Geometry: final body of the model. Coordinates: model frame, mm. Face numbers are marked on the shaded views. A direction names the side the tool comes from. Coordinates: 2 decimals unless noted, no trailing zeros. Write each loop counter-clockwise with the first axis right and the second up, starting at its lowest first coordinate (ties: lowest second). Pieces come first, ordered by that corner, then holes. Notation, with made-up numbers: M -37,-10.5 L -1,-10.5 A32 cw -1,22.5 Z; hole C 8,11.5 d4. An arc over 180 degrees is marked long. Write item = value, one per line. Start each with the question number.
Item 1: Reachability of the marked faces 1 and 2 from +Z, -Z, +X, -X, +Y, -Y: full face, straight path, thin tool, end or side. Return the list, or none.
Item 2: First-contact query: pin 1 Ø2 at (x, z) = (-4.5, -1.5) entering from +Y; pin 2 Ø2 at (x, y) = (2.5, 20) entering from -Z; pin 3 Ø2 at (x, y) = (-4.5, 9) entering from +Z; pin 4 Ø5 at (x, z) = (-3, 2) entering from +Y. Flat tips, straight axial feed; report the tip coordinate or a pass-through.
Item 3: Ray query, L1, parallel to Y at x = -3, z = -1; L2, parallel to Y at x = 1.25, z = 4.75; L3, parallel to X at y = 30.5, z = -0.25. Return the intervals inside material, ascending. Write a range as [from, to].
Item 4: Section B-B on y = 39.5. Output: boundary loops of the cut face in (x, z), plus the area to 3 significant figures.
Item 5: Section A-A on x = 0. Output: boundary loops of the cut face in (y, z).
from build123d import *

# Parameters (mm, degrees)
SKETCH1_R           = 4
BOSS_EXTRUDE1_DEPTH = 65
BOSS_EXTRUDE2_DEPTH = 5
FILLET1_R           = 1
FILLET2_R           = 1


with BuildPart() as part:
    # Sketch1 → Boss-Extrude1 (new body)
    with BuildSketch(Plane(origin=(0, 0, 0), x_dir=(1, 0, 0), z_dir=(0, 1, 0))):
        with Locations(Location((0, 0, 0), (0, 0, 270))):
            Circle(SKETCH1_R)
    extrude(amount=BOSS_EXTRUDE1_DEPTH)

    # Sketch2 → Boss-Extrude2 (add)
    with BuildSketch(Plane.XZ):
        Polygon((-3.464101615, -6), (3.464101615, -6), (6.92820323, 0), (3.464101615, 6), (-3.464101615, 6), (-6.92820323, 0), align=None)
    extrude(amount=BOSS_EXTRUDE2_DEPTH)

    # Fillet1
    fillet1_edges = [part.edges().sort_by_distance(p)[0] for p in [
        (0, 65, -4),
    ]]
    fillet(fillet1_edges, radius=FILLET1_R)

    # Fillet2
    fillet2_edges = [part.edges().sort_by_distance(p)[0] for p in [
        (-5.196152423, 0, -3),
        (-6.92820323, -2.5, 0),
        (0, 0, -6),
        (-3.464101615, -2.5, -6),
        (5.196152423, 0, -3),
        (3.464101615, -2.5, -6),
        (5.196152423, 0, 3),
        (6.92820323, -2.5, 0),
        (0, 0, 6),
        (3.464101615, -2.5, 6),
        (-5.196152423, 0, 3),
        (-3.464101615, -2.5, 6),
        (-5.196152423, -5, -3),
        (0, -5, -6),
        (5.196152423, -5, -3),
        (5.196152423, -5, 3),
        (0, -5, 6),
        (-5.196152423, -5, 3),
    ]]
    fillet(fillet2_edges, radius=FILLET2_R)


solid = part.part
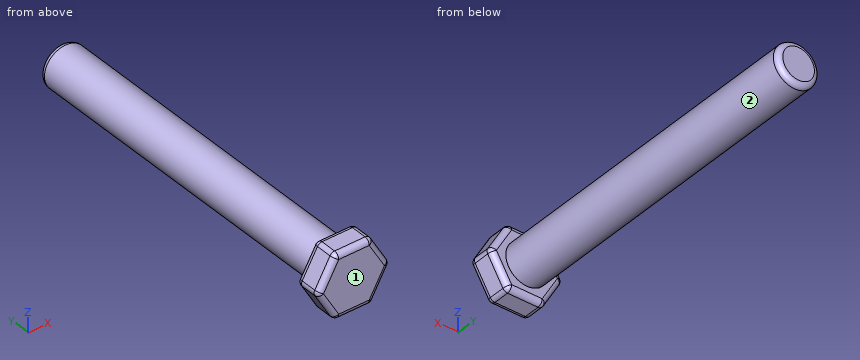
Responses:
q1.face_1 = +Z, -Z, +X, -X, -Y
q1.face_2 = +Y
q2.pin_1 = 64.67
q2.pin_2 = -3.71
q2.pin_3 = 1.94
q2.pin_4 = 65
q3.L1 = [-5, 64.99]
q3.L2 = [-5, 0]
q3.L3 = [-3.99, 3.99]
q4.outline = C 0,0 d8
q4.area = 50.3 mm²
q5.outline = M -5,-5 A1 ccw -4,-6 L -1,-6 A1 ccw 0,-5 L 0,-4 L 64,-4 A1 ccw 65,-3 L 65,3 A1 ccw 64,4 L 0,4 L 0,5 A1 ccw -1,6 L -4,6 A1 ccw -5,5 Z
